The figure shows three views and two pictorial views of one solid part (mm, origin at its lowest corner). Answer the questions. A direction names the side the tool comes from. Give positions to 0.01 mm unless a question says otherwise; leave off trailing zeros. Loops run counter-clockwise (first coordinate to the right, second up) from the corner with the lowest first, then second, coordinate; pieces in that order, holes last. Notation, with made-up numbers: (61, 13.5) - (95, 13.5) arc R12 cw to (95, 34.5) - close; hole circle Ø8 at (40, 65). An arc over 180 degrees is marked (long way). One line per question, with ' | ' between items.
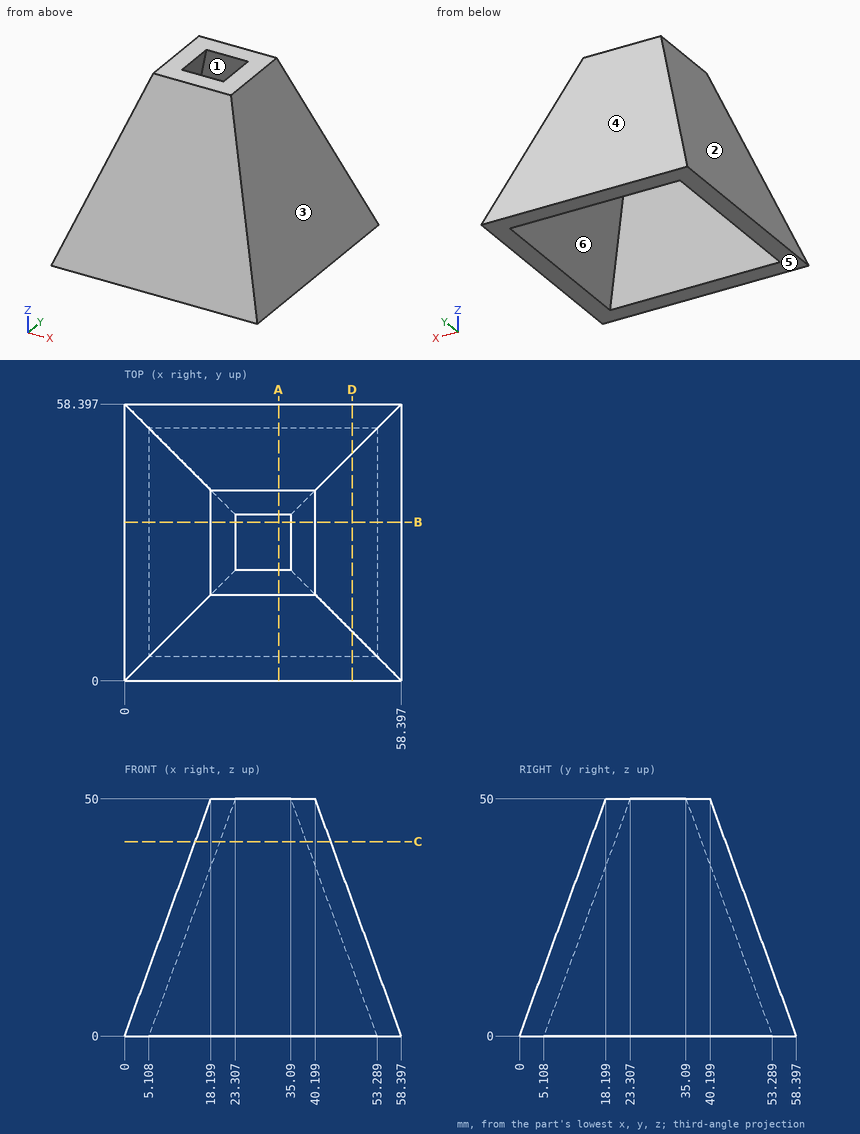
1. Which of the six approach directions +Z, -Z, +X, -X, +Y, -Y give full straight-line access (tool end or side, diameter ignored) to the marked faces 5 and 6?
Evaluation:
face 5: -Z, +X, -X, +Y, -Y | face 6: -Z
2. Determine the mould class of the marked faces 1, 2, 3 and 4 for opening direction X: +X half, -X half, draft (parallel to the pull), parting line (faces both ways), or undercut.
Evaluation:
face 1: undercut | face 2: -X half | face 3: +X half | face 4: draft
3. Find section D-D on x = 48. Write down the section's boundary in (y, z) (1 decimal), then the cut area to 3 significant figures.
Evaluation:
outline: (0, 0) - (5.1, 0) - (10.4, 14.5) - (48, 14.5) - (53.3, 0) - (58.4, 0) - (48, 28.6) - (10.4, 28.6) - close | area: 748 mm2
4. Consider L1, parallel to Y at x = 28, z = 6.5 (1 decimal); L2, parallel to Y at x = 35, z = 28 (1 decimal); L3, parallel to X at y = 29.5, z = 37 (1 decimal). Determine where each line is inside the solid, lowest interval first.
Evaluation:
L1: 2.4 to 7.5, 50.9 to 56 | L2: 10.2 to 15.3, 43.1 to 48.2 | L3: 13.5 to 18.6, 39.8 to 44.9
5. Find section C-C on z = 41. Write down the section's boundary in (x, y) (1 decimal).
Evaluation:
outline: (14.9, 14.9) - (43.5, 14.9) - (43.5, 43.5) - (14.9, 43.5) - close; hole (20, 20) - (38.4, 20) - (38.4, 38.4) - (20, 38.4) - close
6. Flat-ended cylindrical pins translate along their axes: pin 1 (1.5 mm diameter, centred on x = 18.5, z = 13.5, fed in from -Y); pin 2 (10 mm diameter, centred on x = 47, z = 21, fed in from +Y); pin 3 (5 mm diameter, centred on x = 19, z = 8, fed in from -Y). Find the tip coordinate at first contact, or state that the pin passes through.
Evaluation:
pin 1: y = 4.64 | pin 2: y = 52.57 | pin 3: y = 2
7. Find section A-A on x = 32.5. Write down the section's boundary in (y, z).
Evaluation:
outline: (0, 0) - (5.11, 0) - (23.31, 50) - (18.2, 50) - close; (35.09, 50) - (53.29, 0) - (58.4, 0) - (40.2, 50) - close
